Autodesk Inventor part; units mm, degrees
ref_plane "YZ Plane" through (0, 0, 0) normal (1, 0, 0) x (0, 1, 0)
ref_plane "XZ Plane" through (0, 0, 0) normal (0, 1, 0) x (-1, 0, 0)
ref_plane "XY Plane" through (0, 0, 0) normal (0, 0, 1) x (1, 0, 0)
sketch "Boceto1" plane through (0, 0, 0) normal (0, 1, 0) x (-1, 0, 0)
  line L0 (50, 50) -> (-50, 50)
  line L1 (-50, 50) -> (-50, -50)
  line L2 (-50, -50) -> (50, -50)
  line L3 (50, -50) -> (50, 50)
  line L4 (50, 50) -> (-50, -50) construction
  line L5 (-50, 50) -> (50, -50) construction
  point P0 (0, 0)
  dimension "d0" = 100
  dimension "d1" = 100
sketch "Boceto2" plane through (0, 0, 0) normal (0, 1, 0) x (-1, 0, 0)
  point P0 (0, 0)
extrude "Extrusión1" add sketch "Boceto1" along normal blind 50
sketch "Boceto3" plane through (0, 50, 0) normal (0, 1, 0) x (1, 0, 0)
  line L0 (-50, 50) -> (-50, -50)
  line L1 (50, 50) -> (-50, 50)
  line L2 (50, -50) -> (50, 50)
  line L3 (-50, -50) -> (50, -50)
  point P0 (0, 0)
  point P1 (-45, -45)
  point P2 (-45, 45)
  point P3 (45, 45)
  point P4 (45, -45)
  dimension "d11" = 5
  dimension "d12" = 5
  dimension "d13" = 5
  dimension "d14" = 5
  dimension "d15" = 5
  dimension "d16" = 5
  dimension "d17" = 5
  dimension "d18" = 5
hole "Agujero1" at (-45, 50, 45) at (-45, 50, -45) at (45, 50, -45) at (45, 50, 45) direction (0, -1, 0) diameter 6.917 end through all counterbore diameter 8 counterbore depth 0
fillet "Empalme1" radius 5 4 edges at (-50, 25, 50) (50, 25, 50) (50, 25, -50) (-50, 25, -50)
sketch "Boceto4" plane through (0, 50, 0) normal (0, 1, 0) x (1, 0, 0)
  point P0 (0, 0)
sketch "Boceto5" plane through (0, 50, 0) normal (0, 1, 0) x (1, 0, 0)
  circle A0 centre (0, 0) radius 35
  dimension "d20" = 70
extrude "Extrusión2" add sketch "Boceto5" along normal blind 50
fillet "Empalme2" radius 5 1 edges at (-35, 100, 0)
sketch "Boceto7" plane through (0, 100, 0) normal (0, 1, 0) x (1, 0, 0)
  point P0 (0, 0)
hole "Agujero3" at (0, 100, 0) direction (0, -1, 0) diameter 45.6699 depth 30 counterbore diameter 50 counterbore depth 0
properties part number "Practica1Inventor"
CAD build for the part. Positions are in the model's coordinates, mm. A direction names the side the tool comes from. Coordinates: 2 decimals unless noted, no trailing zeros. Order: outer loops, then holes, each group sorted by start corner. A loop starts at its lowest first (then second) coordinate and runs counter-clockwise, first axis right, second up. Notation, with made-up numbers: (56.25, -35) -> (103.25, -35) arc R30 cw to (103.25, 2) -> close; hole circle Ø7 at (85.25, -27). An arc over 180 degrees is marked (long way). Use one line per item in the form item = value. Start each with the question number.
1) Drop flat-ended pins along their axis: pin 1 (3 mm diameter, centred on y = 76, z = 2, fed in from +X); pin 2 (2 mm diameter, centred on x = -33.5, z = 11, fed in from +Y); pin 3 (13.5 mm diameter, centred on x = 2, z = 8.5, fed in from +Y). Give the stop position or say it passes through.
2) Band-saw the part on A-A on y = 31. Give the cut face in (x, z), then the cut area to 3 significant figures.
3) Pull direction Z, two halves, no side cores. Call faces 3 (the cylindrical face through (48.376, 24.65, 44.25)), 4 (the cylindrical face through (-41.624, 24.65, 44.25)), 5 (the cylindrical face through (-49, 25, 48)), 6 (the flat face through (34, 50, 12)): +Z half, -Z half, draft (parallel to the pull), parting line (faces both ways), or undercut.
4) Tool access for faces 1 (the cylindrical face through (-28, 72, -21)), 2 (the flat face through (-50, 25, -1)): list every direction of +Z, -Z, +X, -X, +Y, -Y with a clear straight run to the whole face (end or side of a thin tool).
5) Band-saw the part on D-D on y = 79. Give the cut face in (x, z), then the cut area to 3 significant figures.
6) Band-saw the part on B-B on x = 0. Give the cut face in (y, z).
7) Band-saw the part on C-C on z = 0. Give the cut face in (x, y).
8) Drill centre lines: L1, parallel to X at y = 14, z = -45; L2, parallel to Z at x = 0, y = 80. Where is each one in solid material? Low to high. Write a range as [from, to].
Entries:
q1.pin_1 = 35
q1.pin_2 = 97.62
q1.pin_3 = 70
q2.outline = (-50, -45) arc R5 ccw to (-45, -50) -> (45, -50) arc R5 ccw to (50, -45) -> (50, 45) arc R5 ccw to (45, 50) -> (-45, 50) arc R5 ccw to (-50, 45) -> close; hole circle Ø6.92 at (-45, -45); hole circle Ø6.92 at (-45, 45); hole circle Ø6.92 at (45, -45); hole circle Ø6.92 at (45, 45)
q2.area = 9,830 mm2
q3.face_3 = undercut
q3.face_4 = undercut
q3.face_5 = +Z half
q3.face_6 = draft
q4.face_1 = +Y
q4.face_2 = +Z, -Z, -X, +Y, -Y
q5.outline = circle Ø70 at (0, 0); hole circle Ø45.67 at (0, 0)
q5.area = 2,210 mm2
q6.outline = (0, -50) -> (50, -50) -> (50, -35) -> (95, -35) arc R5 ccw to (100, -30) -> (100, -22.83) -> (70, -22.83) -> (70, 22.83) -> (100, 22.83) -> (100, 30) arc R5 ccw to (95, 35) -> (50, 35) -> (50, 50) -> (0, 50) -> close
q7.outline = (-50, 0) -> (50, 0) -> (50, 50) -> (35, 50) -> (35, 95) arc R5 ccw to (30, 100) -> (22.83, 100) -> (22.83, 70) -> (-22.83, 70) -> (-22.83, 100) -> (-30, 100) arc R5 ccw to (-35, 95) -> (-35, 50) -> (-50, 50) -> close
q8.L1 = [-50, -48.46], [-41.54, 41.54], [48.46, 50]
q8.L2 = [-35, -22.83], [22.83, 35]
